```python
from build123d import *

# Parameters (mm, degrees)
BOSS_EXTRUDE1_DEPTH = 3.175
SKETCH3_R           = 1.5875
CUT_EXTRUDE1_DEPTH  = 3.175


with BuildPart() as part:
    # Sketch2 → Boss-Extrude1 (new body)
    with BuildSketch(Plane(origin=(0, 0, 0), x_dir=(1, 0, 0), z_dir=(0, 1, 0))):
        with BuildLine():
            ThreePointArc((36.339836195, 0.843949489), (2.357673267, 11.966979488), (-31.62448966, 0.843949489))
            ThreePointArc((-31.62448966, 0.843949489), (-32.436771272, -4.432657977), (-27.160163805, -5.244939588))
            ThreePointArc((-27.160163805, -5.244939588), (2.357673267, 4.416828792), (31.87551034, -5.244939588))
            ThreePointArc((31.87551034, -5.244939588), (37.152117806, -4.432657977), (36.339836195, 0.843949489))
        make_face()
    extrude(amount=BOSS_EXTRUDE1_DEPTH)

    # Sketch3 → Cut-Extrude1 (cut)
    with BuildSketch(Plane(origin=(0, 3.175, 0), x_dir=(1, 0, 0), z_dir=(0, 1, 0))):
        with Locations((-29.392326733, -2.20049505)):
            Circle(SKETCH3_R)
        with Locations((34.107673267, -2.20049505)):
            Circle(SKETCH3_R)
    extrude(amount=-CUT_EXTRUDE1_DEPTH, mode=Mode.SUBTRACT)


solid = part.part
```
For this review, take the finished solid that the model builds, in its own axes (mm). Coordinates: 2 decimals unless noted, no trailing zeros. Loops run counter-clockwise (first coordinate to the right, second up) from the corner with the lowest first, then second, coordinate; pieces in that order, holes last.
1. Add section A-A, the plane z = -3.5. Give the boundary of the cut face in (x, y) (3 decimals).
2. For line 1 (X direction, y = 2.1, z = 0.75); line 2 (X direction, y = 1.9, z = 1); line 3 (X direction, y = 1.5, z = -0.5), list the stretches that pass through material, from the lowest coordinate up.
3. Add section C-C, the plane x = -16. Give the boundary of the cut face in (y, z) (3 decimals).
4. Mouldability with a two-part tool opening along X and no side actions: class faces 1 (the flat face through (2, 0, -5)), 2 (the cylindrical face through (-32.485, 1.565, 4.365)), 3 (the cylindrical face through (2.867, 1.565, -11.965)) as +X half, -X half, draft (parallel to the pull), parting line (faces both ways), or undercut.
Result:
1. outline: (-27.668, 0) - (-7.166, 0) - (-7.166, 3.175) - (-27.668, 3.175) - close; (11.881, 0) - (32.383, 0) - (32.383, 3.175) - (11.881, 3.175) - close
2. line 1: x = -32.88 to -30.04, -28.75 to -19.76, 24.47 to 33.46, 34.75 to 37.59
2. line 2: x = -32.97 to -30.43, -28.35 to -20.26, 24.97 to 33.07, 35.15 to 37.69
2. line 3: x = -32.03 to -17.03, 21.74 to 36.75
3. outline: (0, -8.956) - (3.175, -8.956) - (3.175, -0.919) - (0, -0.919) - close
4. face 1: draft
4. face 2: undercut
4. face 3: parting line
